Build history of the part. All positions in model axes, mm. Face numbers are marked on the shaded views. A direction names the side the tool comes from. Give positions to 0.01 mm unless a question says otherwise; leave off trailing zeros. Loops run counter-clockwise (first coordinate to the right, second up) from the corner with the lowest first, then second, coordinate; pieces in that order, holes last.
1) Two-plate mould, pull along X, no slides. Class the marked faces 3, 4 and 5: +X half, -X half, draft (parallel to the pull), parting line (faces both ways), or undercut.
2) 3-axis set-ups, long thin cutter, end or side, ignore diameter. For the marked faces 1 and 2: which of +Z, -Z, +X, -X, +Y, -Y reach the whole face in a straight line?
3) Flat gauge pin, fed straight in: P1, Ø1, axis at x = -0.5, z = 0.5, coming from the +Y side. Where does the tip first touch, or does it go through?
4) Band-saw the part on A-A on y = 16. List the corners of the cut face in (x, z), then the cut area to 3 significant figures.
5) Band-saw the part on B-B on x = 5. List the corners of the cut face in (y, z), then the cut area to 3 significant figures.
6) Band-saw the part on C-C on z = 45. List the corners of the cut face in (x, y), then the cut area to 3 significant figures.
7) Wall check: line 1 (Z direction, x = 0, y = 24.75); line 2 (X direction, y = 0.5, z = 8.5); line 3 (Y direction, x = -9.5, z = -54.5). Give the ranges that are in metal, low to high.
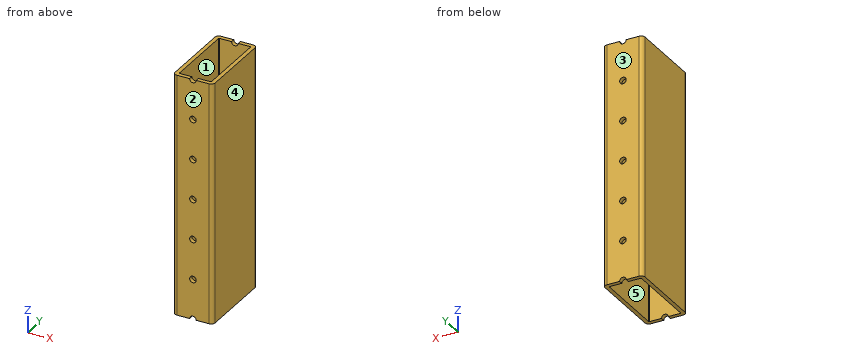
```python
from build123d import *

# Parameters (mm, degrees)
SKETCH1_W                 = 152.4
SKETCH1_H                 = 50.8
BOSS_EXTRUDE1_DEPTH       = 25.4
SKETCH2_W                 = 20.32
SKETCH2_H                 = 45.72
CUT_EXTRUDE1_DEPTH        = 153.4
F_6_CLEARANCE_HOLE1_D     = 4.1402
F_6_CLEARANCE_HOLE1_DEPTH = 50.8
F_6_CLEARANCE_HOLE2_D     = 4.1402
F_6_CLEARANCE_HOLE2_DEPTH = 50.8
FILLET1_R                 = 0.5
FILLET2_R                 = 2.54


with BuildPart() as part:
    # Sketch1 → Boss-Extrude1 (new body)
    with BuildSketch(Plane(origin=(12.7, 0, 0), x_dir=(0, 0, -1), z_dir=(1, 0, 0))):
        Rectangle(SKETCH1_W, SKETCH1_H)
    extrude(amount=-BOSS_EXTRUDE1_DEPTH)

    # Sketch2 → Cut-Extrude1 (cut, through all)
    with BuildSketch(Plane(origin=(0, 0, -76.2), x_dir=(-1, 0, 0), z_dir=(0, 0, -1))):
        Rectangle(SKETCH2_W, SKETCH2_H)
    extrude(amount=-CUT_EXTRUDE1_DEPTH, mode=Mode.SUBTRACT)

    # #6 Clearance Hole1
    with Locations(Plane(origin=(0, -25.4, 0), x_dir=(-1, 0, 0), z_dir=(0, -1, 0))):
        with Locations((0, 711.2), (0, 736.6), (0, 685.8), (0, 660.4), (0, 635), (0, 609.6), (0, 584.2), (0, 558.8), (0, 533.4), (0, 508), (0, 482.6), (0, 457.2), (0, 431.8), (0, 406.4), (0, 381), (0, 355.6), (0, 330.2), (0, 304.8), (0, 279.4), (0, 254), (0, 228.6), (0, 203.2), (0, 177.8), (0, 152.4), (0, 127), (0, 101.6), (0, 76.2), (0, 50.8), (0, 25.4), (0, 0), (0, -25.4), (0, -50.8), (0, -76.2), (0, -101.6), (0, -127), (0, -152.4), (0, -177.8), (0, -203.2), (0, -228.6), (0, -254), (0, -279.4), (0, -304.8), (0, -330.2), (0, -355.6), (0, -381), (0, -406.4), (0, -431.8), (0, -457.2), (0, -482.6), (0, -508), (0, -533.4), (0, -558.8), (0, -584.2), (0, -609.6), (0, -635), (0, -660.4), (0, -685.8), (0, -711.2), (0, -736.6)):
            Hole(F_6_CLEARANCE_HOLE1_D / 2, depth=F_6_CLEARANCE_HOLE1_DEPTH)

    # #6 Clearance Hole2
    with Locations(Plane(origin=(0, 25.4, 0), x_dir=(1, 0, 0), z_dir=(0, 1, 0))):
        with Locations((0, 711.2), (0, 736.6), (0, 685.8), (0, 660.4), (0, 635), (0, 609.6), (0, 584.2), (0, 558.8), (0, 533.4), (0, 508), (0, 482.6), (0, 457.2), (0, 431.8), (0, 406.4), (0, 381), (0, 355.6), (0, 330.2), (0, 304.8), (0, 279.4), (0, 254), (0, 228.6), (0, 203.2), (0, 177.8), (0, 152.4), (0, 127), (0, 101.6), (0, 76.2), (0, 50.8), (0, 25.4), (0, 0), (0, -25.4), (0, -50.8), (0, -76.2), (0, -101.6), (0, -127), (0, -152.4), (0, -177.8), (0, -203.2), (0, -228.6), (0, -254), (0, -279.4), (0, -304.8), (0, -330.2), (0, -355.6), (0, -381), (0, -406.4), (0, -431.8), (0, -457.2), (0, -482.6), (0, -508), (0, -533.4), (0, -558.8), (0, -584.2), (0, -609.6), (0, -635), (0, -660.4), (0, -685.8), (0, -711.2), (0, -736.6)):
            Hole(F_6_CLEARANCE_HOLE2_D / 2, depth=F_6_CLEARANCE_HOLE2_DEPTH)

    # Fillet1
    fillet1_edges = [part.edges().sort_by_distance(p)[0] for p in [
        (-10.16, -22.86, 0),
        (10.16, -22.86, 0),
        (10.16, 22.86, 0),
        (-10.16, 22.86, 0),
    ]]
    fillet(fillet1_edges, radius=FILLET1_R)

    # Fillet2
    fillet2_edges = [part.edges().sort_by_distance(p)[0] for p in [
        (-12.7, 25.4, 0),
        (-12.7, -25.4, 0),
        (12.7, 25.4, 0),
        (12.7, -25.4, 0),
    ]]
    fillet(fillet2_edges, radius=FILLET2_R)


solid = part.part
```
Findings below:
1. face 3: draft
1. face 4: +X half
1. face 5: undercut
2. face 1: +Z, -Z
2. face 2: +Z, -Z, +X, -X, -Y
3. P1: passes through
4. outline: (-12.7, -76.2) - (-10.16, -76.2) - (-10.16, 76.2) - (-12.7, 76.2) - close; (10.16, -76.2) - (12.7, -76.2) - (12.7, 76.2) - (10.16, 76.2) - close
4. area: 774 mm2
5. outline: (-25.4, -76.2) - (-22.86, -76.2) - (-22.86, 76.2) - (-25.4, 76.2) - close; (22.86, -76.2) - (25.4, -76.2) - (25.4, 76.2) - (22.86, 76.2) - close
5. area: 774 mm2
6. outline: (-12.7, -22.86) arc R2.54 ccw to (-10.16, -25.4) - (10.16, -25.4) arc R2.54 ccw to (12.7, -22.86) - (12.7, 22.86) arc R2.54 ccw to (10.16, 25.4) - (-10.16, 25.4) arc R2.54 ccw to (-12.7, 22.86) - close; hole (-10.16, -22.36) arc R0.5 ccw to (-9.66, -22.86) - (9.66, -22.86) arc R0.5 ccw to (10.16, -22.36) - (10.16, 22.36) arc R0.5 ccw to (9.66, 22.86) - (-9.66, 22.86) arc R0.5 ccw to (-10.16, 22.36) - close
6. area: 356 mm2
7. line 1: z = -74.13 to -52.87, -48.73 to -27.47, -23.33 to -2.07, 2.07 to 23.33, 27.47 to 48.73, 52.87 to 74.13
7. line 2: x = -12.7 to -10.16, 10.16 to 12.7
7. line 3: y = -25.4 to -22.86, 22.86 to 25.4
